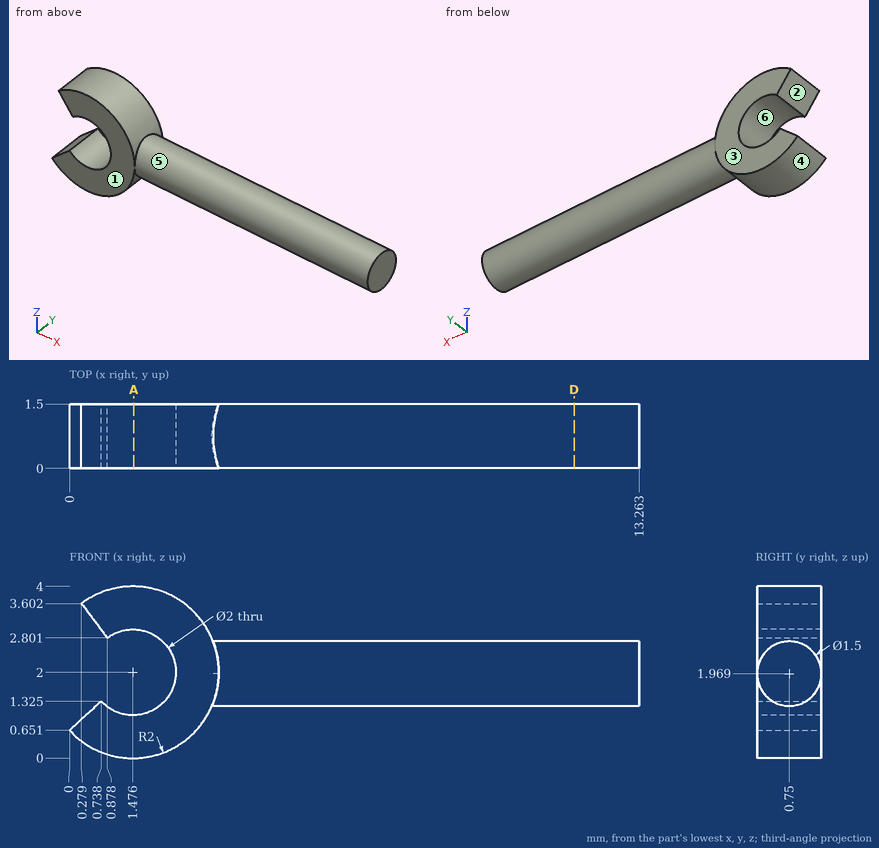
Job drawing, mm, ordinate dimensions from the low corner. One solid piece. A direction names the side the tool comes from. Round coordinates to 2 decimals unless told otherwise and drop trailing zeros. Loops run counter-clockwise (first coordinate to the right, second up) from the corner with the lowest first, then second, coordinate; pieces in that order, holes last.
(1) Two-plate mould, pull along Z, no slides. Class the marked faces 3, 4, 5 and 6: +Z half, -Z half, draft (parallel to the pull), parting line (faces both ways), or undercut.
(2) Wall check: line 1 along X through (y, z) = (0.85, 2); line 2 along Z through (x, y) = (0.5, 0.4) (1 decimal); line 3 along Z through (x, y) = (3.75, 0.9) (1 decimal). Give the ranges that are in metal, low to high.
(3) Cut at A-A (x = 1.5). Give the cut face in (y, z).
(4) Cut at D-D (x = 11.75). Give the cut face in (y, z).
(5) Which spindle directions (+Z, -Z, +X, -X, +Y, -Y) get a long thin tool onto all of the face, cutting with end or side? Do the marked faces 1 and 2. Say none if no direction does.
Findings below:
1. face 3: draft
1. face 4: -Z half
1. face 5: parting line
1. face 6: undercut
2. line 1: x = 2.48 to 13.26
2. line 2: z = 0.3 to 1.1, 3.3 to 3.7
2. line 3: z = 1.2 to 2.7
3. outline: (0, 0) - (1.5, 0) - (1.5, 1) - (0, 1) - close; (0, 3) - (1.5, 3) - (1.5, 4) - (0, 4) - close
4. outline: circle Ø1.5 at (0.75, 1.97)
5. face 1: +Z, -Z, +X, -X, -Y
5. face 2: -X, +Y, -Y
